from build123d import *

# Parameters (mm, degrees)
BOSS_EXTRUDE1_DEPTH      = 5.5
BOSS_EXTRUDE1_DEPTH_BACK = 5.5
SKETCH1_R                = 1.6
SKETCH4_R                = 3
CUT_EXTRUDE2_DEPTH       = 5
BOSS_EXTRUDE2_DEPTH      = 11
FILLET1_R                = 0.4
SKETCH7_R                = 0.95
CUT_EXTRUDE3_DEPTH       = 30.124654232
CUT_EXTRUDE5_DEPTH       = 10
CUT_EXTRUDE5_DEPTH_BACK  = 30.124654236
CUT_EXTRUDE5_START       = -18.97961
SKETCH8_R                = 2.1
FILLET2_R                = 5
SKETCH9_R                = 3.25
CUT_EXTRUDE6_DEPTH       = 8
BOSS_EXTRUDE3_START      = -11
SKETCH10_W               = 5.65
SKETCH10_H               = 9.7
BOSS_EXTRUDE3_DEPTH      = 11
SKETCH11_R               = 3.7
CUT_EXTRUDE7_DEPTH       = 3
FILLET3_R                = 5


with BuildPart() as part:
    # Sketch1 → Boss-Extrude1 (new, two sides: drawn at the far end of the back side and taken through both)
    with BuildSketch(Plane.XY.offset(-BOSS_EXTRUDE1_DEPTH_BACK)):
        with BuildLine():
            Line((-15.5, 5.65), (15.5, 5.65))
            ThreePointArc((15.5, 5.65), (21.15, 0), (15.5, -5.65))
            Line((15.5, -5.65), (-15.5, -5.65))
            ThreePointArc((-15.5, -5.65), (-21.15, 0), (-15.5, 5.65))
        make_face()
        with Locations((-15.5, 0)):
            Circle(SKETCH1_R, mode=Mode.SUBTRACT)
        with Locations(Location((15.5, 0, 0), (0, 0, 180))):
            Circle(SKETCH1_R, mode=Mode.SUBTRACT)
    extrude(amount=BOSS_EXTRUDE1_DEPTH + BOSS_EXTRUDE1_DEPTH_BACK)

    # Sketch4 → Cut-Extrude2 (cut)
    with BuildSketch(Plane(origin=(0, 5.65, 0), x_dir=(1, 0, 0), z_dir=(0, 1, 0))):
        with Locations(Location((6.375, 0, 0), (0, 0, 180))):
            Circle(SKETCH4_R)
    extrude(amount=-CUT_EXTRUDE2_DEPTH, mode=Mode.SUBTRACT)

    # Sketch6 → Boss-Extrude2 (add)
    with BuildSketch(Plane.XY.offset(5.5)):
        with BuildLine():
            Line((-0.65013639, -9.535327111), (-0.65013639, -5.65))
            Line((-0.65013639, -5.65), (13.939015195, -5.65))
            Line((13.939015195, -5.65), (13.939015195, -8.737119999))
            ThreePointArc((13.939015195, -8.737119999), (8.407998992, -10.285488801), (6, -15.5))
            ThreePointArc((6, -15.5), (4.006194058, -11.03341191), (-0.65013639, -9.535327111))
        make_face()
    extrude(amount=-BOSS_EXTRUDE2_DEPTH)

    # Fillet1
    fillet1_edges = [part.edges().sort_by_distance(p)[0] for p in [
        (6, -15.5, 0),
    ]]
    fillet(fillet1_edges, radius=FILLET1_R)

    # Sketch7 → Cut-Extrude3 (cut, through all)
    with BuildSketch(Plane(origin=(0, 5.65, 0), x_dir=(1, 0, 0), z_dir=(0, 1, 0))):
        with Locations(Location((6.375, 0, 0), (0, 0, 180))):
            Circle(SKETCH7_R)
    extrude(amount=-CUT_EXTRUDE3_DEPTH, mode=Mode.SUBTRACT)

    # Sketch8 → Cut-Extrude5 (cut, two sides: drawn at the far end of the back side and taken through both)
    with BuildSketch(Plane(origin=(0, 5.65, 0), x_dir=(1, 0, 0), z_dir=(0, 1, 0)).offset(CUT_EXTRUDE5_START - CUT_EXTRUDE5_DEPTH_BACK)):
        with Locations(Location((6.375, 0, 0), (0, 0, 180))):
            Circle(SKETCH8_R)
    extrude(amount=CUT_EXTRUDE5_DEPTH + CUT_EXTRUDE5_DEPTH_BACK, mode=Mode.SUBTRACT)

    # Fillet2
    # the kernel refuses this fillet: 5 mm, written as the material it adds along each edge
    with BuildSketch(Plane(origin=(13.939015195, -5.65, 5.5), x_dir=(0, -1, 0), z_dir=(0, 0, -1))) as fillet2_piece_1:
        with BuildLine():
            CenterArc((4.496369398, -4.797292583), FILLET2_R, 106.370642389, 55.938643206)
            Line((-0.26718431, -3.27789926), (-0.743539681, -3.125959928))
            ThreePointArc((-0.743539681, -3.125959928), (-0.5, -1.560984805), (-0.5, 0))
            Line((-0.5, 0), (0, 0.5))
            ThreePointArc((0, 0.5), (1.54356, 0.5), (2.946195059, 0.479729258))
            Line((2.946195059, 0.479729258), (3.087119999, 0))
        make_face()
    extrude(amount=11)
    with BuildSketch(Plane(origin=(-0.65013639, -5.65, 5.5), x_dir=(0, -1, 0), z_dir=(0, 0, -1))) as fillet2_piece_2:
        with BuildLine():
            CenterArc((5, 4.874167042), FILLET2_R, 180, 77.118546425)
            Line((0, 4.874167042), (-0.1, 4.874167042))
            Line((-0.1, 4.874167042), (-0.1, 0))
            Line((-0.1, 0), (0, -0.1))
            ThreePointArc((0, -0.1), (1.942663555, -0.1), (3.863033653, -0.097483341))
            Line((3.863033653, -0.097483341), (3.885327111, 0))
        make_face()
    extrude(amount=11)

    # Sketch9 → Cut-Extrude6 (cut)
    with BuildSketch(Plane.XY.offset(5.5)):
        with Locations((-15.5, 0)):
            Circle(SKETCH9_R)
        with Locations((15.5, 0)):
            Circle(SKETCH9_R)
    extrude(amount=-CUT_EXTRUDE6_DEPTH, mode=Mode.SUBTRACT)

    # Sketch10 → Boss-Extrude3 (add)
    with BuildSketch(Plane.XY.offset(5.5).offset(BOSS_EXTRUDE3_START)):
        with Locations((-12.675, -10.5)):
            Rectangle(SKETCH10_W, SKETCH10_H)
        with BuildLine():
            Line((-15.5, -15.35), (-15.5, -5.65))
            ThreePointArc((-15.5, -5.65), (-19.495153314, -3.995153314), (-21.15, 0))
            Line((-21.15, 0), (-21.15, -15.35))
            Line((-21.15, -15.35), (-15.5, -15.35))
        make_face()
    extrude(amount=BOSS_EXTRUDE3_DEPTH)

    # Sketch11 → Cut-Extrude7 (cut)
    with BuildSketch(Plane.XZ.offset(15.35)):
        with Locations(Location((-15.5, 0, 0), (0, 0, 270))):
            Circle(SKETCH11_R)
    extrude(amount=-CUT_EXTRUDE7_DEPTH, mode=Mode.SUBTRACT)

    # Fillet3
    # the kernel refuses this fillet: 5 mm, written as the material it adds along each edge
    with BuildSketch(Plane(origin=(-9.85, -5.65, -5.5), x_dir=(1, 0, 0), z_dir=(0, 0, 1))) as fillet3_piece_1:
        with BuildLine():
            CenterArc((5, -4.954322848), FILLET3_R, 97.75056413, 82.24943587)
            Line((0, -4.954322848), (-0.1, -4.954322848))
            Line((-0.1, -4.954322848), (-0.1, 0))
            Line((-0.1, 0), (0, 0.1))
            ThreePointArc((0, 0.1), (2.162848284, 0.1), (4.3122105, 0.099086457))
            Line((4.3122105, 0.099086457), (4.325696569, 0))
        make_face()
    extrude(amount=11)


solid = part.part
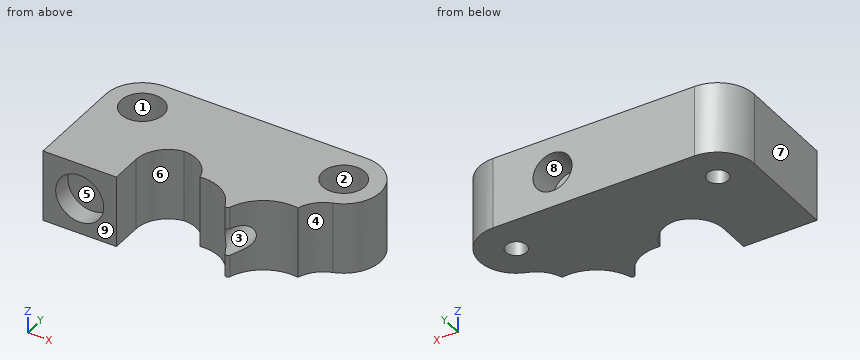
Could you check a few things on this model? Use its own coordinates, in mm. Face numbers are marked on the shaded views. A direction names the side the tool comes from. Give positions to 0.01 mm unless a question says otherwise; leave off trailing zeros. Order: outer loops, then holes, each group sorted by start corner. A loop starts at its lowest first (then second) coordinate and runs counter-clockwise, first axis right, second up. Notation, with made-up numbers: (48.5, 27.5) - (73.5, 27.5) arc R21 cw to (73.5, 60.5) - close; hole circle Ø11 at (-9.5, -27.5). An arc over 180 degrees is marked (long way). Return JSON: item names as keys, results as strings. Group by question number.
Q1. Suppose I cut it at D-D, the plane z = 4.25. State how many separate pieces and enclosed holes the cut face has, and give its area (3 significant figures).
Q2. Suppose I cut it at C-C, the plane x = -18. Please give me the cut outline in (y, z), and give its area (3 significant figures).
Q3. Suppose I cut it at A-A, the plane y = -0.5. Please give me the cut outline in (x, z) (3 decimals).
Q4. Suppose I cut it at B-B, the plane z = 0. Please give me the cut outline in (x, y) (3 decimals).
Q5. Thinking about a two-plate mould opening in Y: for the marked faces 1, 2, 3 and 4, which applies, pulls with the +Y half, pulls with the -Y half, needs draft (parallel to the pull), parting line crosses it, or undercut?
Q6. Will these pins go through, and if not, where does the flat tip stop? pin 1 Ø3 at (x, y) = (15.5, 0) entering from +Z; pin 2 Ø1.5 at (x, z) = (16, -0.5) entering from -Y; pin 3 Ø2 at (x, z) = (-15, 0) entering from -Y; pin 4 Ø4 at (y, z) = (-14, -1.5) entering from +X.
Q7. Which directions (+Z, -Z, +X, -X, +Y, -Y) give clear straight access to the entire face, cutting with the end or side of a thin tool? Please do the marked faces 5, 6, 7, 8 and 9.
Q8. Please list where these lines run through material, in increasing order: line 1 along X through (y, z) = (-8.5, 0) (3 decimals); line 2 along X through (y, z) = (0.5, 4); line 3 along X through (y, z) = (-14.25, 4.5). Write a range as [from, to].
Resolved:
{
 "1": {"separate pieces": "1", "enclosed holes": "2", "area": "580 mm2"},
 "2": {"outline": "(-15.35, -5.5) - (5.07, -5.5) - (5.07, 5.5) - (2.08, 5.5) - (2.08, -2.5) - (-2.08, -2.5) - (-2.08, 5.5) - (-15.35, 5.5) - (-15.35, 2.73) - (-12.35, 2.73) - (-12.35, -2.73) - (-15.35, -2.73) - close", "area": "175 mm2"},
 "3": {"outline": "(-21.15, -5.5) - (-17.02, -5.5) - (-17.02, -2.5) - (-18.711, -2.5) - (-18.711, 5.5) - (-21.15, 5.5) - close; (-13.98, -5.5) - (13.98, -5.5) - (13.98, -2.5) - (12.289, -2.5) - (12.289, 5.5) - (-12.289, 5.5) - (-12.289, -2.5) - (-13.98, -2.5) - close; (17.02, -5.5) - (21.128, -5.5) - (21.128, 5.5) - (18.711, 5.5) - (18.711, -2.5) - (17.02, -2.5) - close; hole circle Ø1.9 at (6.375, 0)"},
 "4": {"outline": "(-21.15, -15.35) - (-19.2, -15.35) - (-19.2, -12.35) - (-11.8, -12.35) - (-11.8, -15.35) - (-9.85, -15.35) - (-9.85, -10.604) arc R5 cw to (-5.524, -5.65) arc R5 cw to (-0.65, -9.535) arc R6 cw to (4.275, -11.29) - (4.275, -3.33) - (5.425, -3.33) - (5.425, 0.65) - (3.375, 0.65) - (3.375, 5.65) - (-15.5, 5.65) arc R5.65 ccw to (-21.15, 0) - close; (7.325, -3.33) - (8.475, -3.33) - (8.475, -10.229) arc R6.85 cw to (13.939, -8.737) arc R5 cw to (17.217, -5.383) arc R5.65 ccw to (15.5, 5.65) - (9.375, 5.65) - (9.375, 0.65) - (7.325, 0.65) - close; hole circle Ø6.5 at (-15.5, 0); hole circle Ø6.5 at (15.5, 0)"},
 "5": {"face 1": "undercut", "face 2": "undercut", "face 3": "needs draft", "face 4": "pulls with the -Y half"},
 "6": {"pin 1": "passes through", "pin 2": "stops at y = -6.56", "pin 3": "stops at y = -12.35", "pin 4": "stops at x = 6.92"},
 "7": {"face 5": "-Y", "face 6": "+Z, -Z, -Y", "face 7": "+Z, -Z, -X, +Y, -Y", "face 8": "+Y", "face 9": "+Z, -Z, +X, -X, -Y"},
 "8": {"line 1": "x = [-21.15, -9.386], [-1.01, 4.275], [8.475, 14.015]", "line 2": "x = [-21.13, -18.71], [-12.29, 12.29], [18.71, 21.13]", "line 3": "x = [-21.15, -9.85]"}
}
